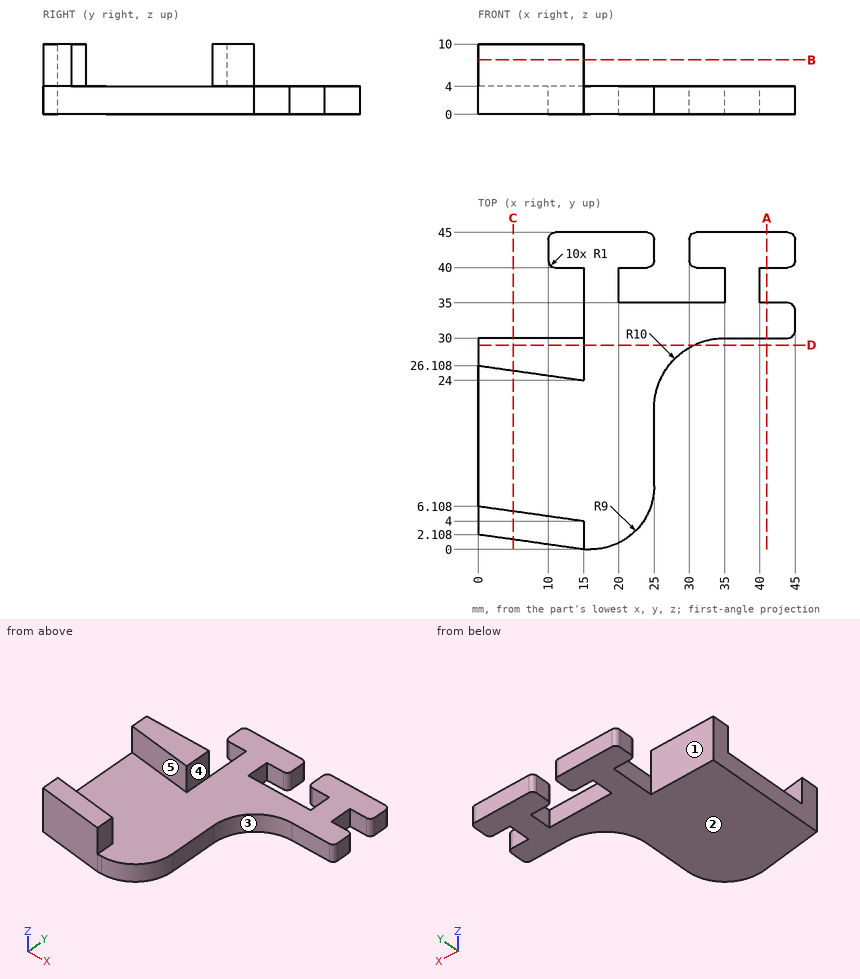
Drawing for the job (mm, zero at the part's lowest x, y, z). A direction names the side the tool comes from. Coordinates: 2 decimals unless noted, no trailing zeros. Loops run counter-clockwise (first coordinate to the right, second up) from the corner with the lowest first, then second, coordinate; pieces in that order, holes last. Notation, with made-up numbers: (15.25, 87) - (29.25, 87) arc R23 cw to (29.25, 97) - close; hole circle Ø10 at (87, 51). An arc over 180 degrees is marked (long way). Use CSV: the item, a comma, the result in double quotes. Start each with the question number.
Q1. Cut at C-C, the plane x = 5. List the corners of the cut face in (y, z).
Q2. Cut at D-D, the plane y = 29. List the corners of the cut face in (x, z).
Q3. Drop flat-ended pins along their axis: P1, Ø1.5, axis at y = 42, z = 2.5, coming from the -X side; P2, Ø2, axis at x = 40.5, z = 2.5, coming from the -Y side; P3, Ø4, axis at x = 34, z = 5.5, coming from the +Y side; P4, Ø1, axis at x = 31.5, z = 1, coming from the -Y side (3 decimals). Give the stop position or say it passes through.
Q4. 3-axis set-ups, long thin cutter, end or side, ignore diameter. For the marked faces 1, 2, 3, 4 and 5: which of +Z, -Z, +X, -X, +Y, -Y reach the whole face in a straight line?
Q5. Probe probe 1 along Z at (x, y) = (7.5, 12.5); probe 2 along X at (y, z) = (20, 2); probe 3 along Y at (x, z) = (3.5, 9.5). List the from-to ranges inside material, lowest first. Write a range as from..to.
Q6. Cut at A-A, the plane x = 41. List the corners of the cut face in (y, z), then the cut area to 3 significant figures.
Q7. Cut at B-B, the plane z = 7.75. List the corners of the cut face in (x, y), then the cut area to 3 significant figures.
Here are the results:
1,outline,"(1.41, 0) - (30, 0) - (30, 10) - (25.41, 10) - (25.41, 4) - (5.41, 4) - (5.41, 10) - (1.41, 10) - close"
2,outline,"(0, 0) - (30.64, 0) - (30.64, 4) - (15, 4) - (15, 10) - (0, 10) - close"
3,P1,"x = 10"
3,P2,"y = 30"
3,P3,"y = 45"
3,P4,"y = 29.165"
4,face 1,"+Z, -Z, -X"
4,face 2,"-Z, +X, -X, +Y, -Y"
4,face 3,"+Z, -Z, +X, -Y"
4,face 4,"+Z, +X, +Y, -Y"
4,face 5,"+Z, -X"
5,probe 1,"0..4"
5,probe 2,"0..25"
5,probe 3,"1.62..5.62, 25.62..30"
6,outline,"(30, 0) - (35, 0) - (35, 4) - (30, 4) - close; (40, 0) - (45, 0) - (45, 4) - (40, 4) - close"
6,area,"40.0 mm2"
7,outline,"(0, 2.11) - (15, 0) - (15, 4) - (0, 6.11) - close; (0, 26.11) - (15, 24) - (15, 30) - (0, 30) - close"
7,area,"134 mm2"
